Part model, mm, in its own coordinate system. Coordinates: 2 decimals unless noted, no trailing zeros. Order: outer loops, then holes, each group sorted by start corner. A loop starts at its lowest first (then second) coordinate and runs counter-clockwise, first axis right, second up.
Autodesk Inventor part; units mm, degrees
ref_plane "YZ Plane" through (0, 0, 0) normal (1, 0, 0) x (0, 1, 0)
ref_plane "XZ Plane" through (0, 0, 0) normal (0, 1, 0) x (-1, 0, 0)
ref_plane "XY Plane" through (0, 0, 0) normal (0, 0, 1) x (1, 0, 0)
sketch "スケッチ1" plane through (0, 0, 0) normal (0, 0, 1) x (1, 0, 0)
  circle A0 centre (0, 0) radius 7.7
  circle A1 centre (0, 0) radius 2.1
  dimension "d0" = 4.2
  dimension "d1" = 15.4
extrude "押し出し1" add sketch "スケッチ1" along normal blind 1
chamfer "面取り1" distance 0.4 angle 45 1 edges at (-7.7, 0, 0)
sketch "スケッチ2" plane through (0, 0, 1) normal (0, 0, 1) x (1, 0, 0)
  circle A0 centre (0, 3.5) radius 0.5915 construction
  point P0 (0, 0)
  point P1 (-3.0311, -1.75)
  point P2 (3.0311, -1.75)
  dimension "d9" = 360
hole "穴1" at (0, 3.5, 1) at (-3.0311, -1.75, 1) at (3.0311, -1.75, 1) direction (0, 0, -1) diameter 1.5 end through all countersink diameter 2.2 countersink angle 82
properties part number "INNER_TIMING_PULLEY_COVER"
Q1. Mould opens along X. For faces 1 (the face through (2, -2, 0)), 2 (the face through (-1.669, 7.517, 0.696)), 3 (the face through (-0.03, 4.25, 0.29)) say: pulls with the +X half, pulls with the -X half, needs draft (parallel to the pull), parting line crosses it, or undercut.
Results list:
face 1: needs draft
face 2: parting line crosses it
face 3: undercut
Q2. Cut at D-D on y = -1.75. Count the separate pieces of the cut face and the enclosed holes in it, and give its area (3 significant figures).
Results list:
separate pieces: 4
enclosed holes: 0
area: 9.23 mm2
Q3. Cut at B-B on y = 0. Write the cut outline in (x, z).
Results list:
outline: (-7.7, 0.4) - (-7.3, 0) - (-2.1, 0) - (-2.1, 1) - (-7.7, 1) - close; (2.1, 0) - (7.3, 0) - (7.7, 0.4) - (7.7, 1) - (2.1, 1) - close
Q4. Cut at C-C on z = 0.2. Write the cut outline in (x, y).
Results list:
outline: circle Ø15 at (0, 0); hole circle Ø1.5 at (-3.03, -1.75); hole circle Ø4.2 at (0, 0); hole circle Ø1.5 at (0, 3.5); hole circle Ø1.5 at (3.03, -1.75)
Q5. Cut at A-A on x = 0. Write the cut outline in (y, z), and give its area (3 significant figures).
Results list:
outline: (-7.7, 0.4) - (-7.3, 0) - (-2.1, 0) - (-2.1, 1) - (-7.7, 1) - close; (2.1, 0) - (2.75, 0) - (2.75, 0.6) - (2.4, 1) - (2.1, 1) - close; (4.25, 0) - (7.3, 0) - (7.7, 0.4) - (7.7, 1) - (4.6, 1) - (4.25, 0.6) - close
area: 9.40 mm2
Q6. Pin check, flat tip, straight feed: pin 1 Ø1.7 at (x, y) = (0, 3.5) entering from -Z. Stop position of the tip, or through.
Results list:
pin 1: stops at z = 0
Q7. Wall check: line 1 along X through (y, z) = (-1.75, 0.25); line 2 along X through (y, z) = (-1.5, 0.1); line 3 along Y through (x, z) = (3.5, 0.65). Give the ranges that are in metal, low to high.
Results list:
line 1: x = -7.34 to -3.78, -2.28 to -1.16, 1.16 to 2.28, 3.78 to 7.34
line 2: x = -7.25 to -3.74, -2.32 to -1.47, 1.47 to 2.32, 3.74 to 7.25
line 3: y = -6.86 to -2.39, -1.11 to 6.86
